Part print with two shaded views. Sizes in mm from the minimum x, y, z corner. Give positions to 0.01 mm unless a question says otherwise; leave off trailing zeros. Order: outer loops, then holes, each group sorted by start corner. A loop starts at its lowest first (then second) coordinate and runs counter-clockwise, first axis right, second up. Notation, with made-up numbers: M 41,3.5 L 46,3.5 A26 cw 46,24.5 Z; hole C -22,19.25 d4. An arc over 180 degrees is marked long. Return JSON: item names as keys, results as strings.
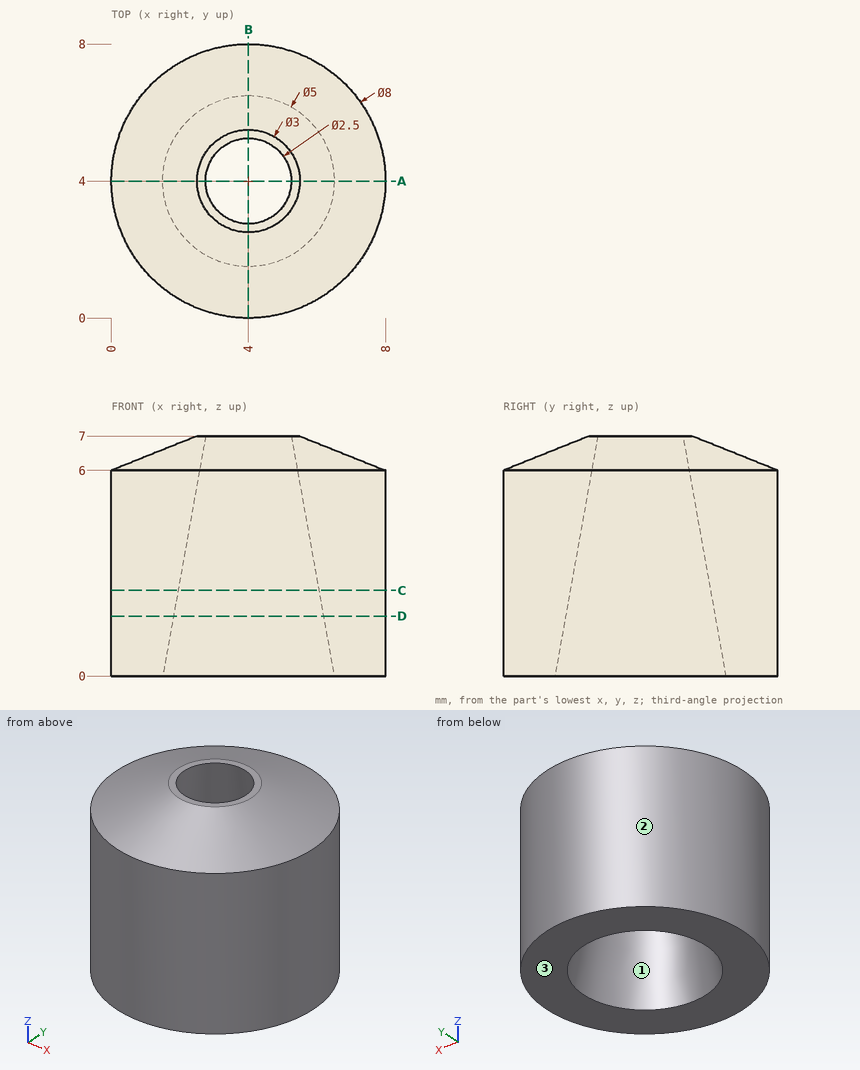
Q1. Two-plate mould, pull along Y, no slides. Class the marked faces 1, 2 and 3: +Y half, -Y half, draft (parallel to the pull), parting line (faces both ways), or undercut.
Established:
{"face 1": "undercut", "face 2": "parting line", "face 3": "draft"}
Q2. Band-saw the part on A-A (y = 4). Give the cut face in (x, z), then the cut area to 4 significant figures.
Established:
{"outline": "M 0,0 L 1.5,0 L 2.75,7 L 2.5,7 L 0,6 Z; M 5.25,7 L 6.5,0 L 8,0 L 8,6 L 5.5,7 Z", "area": "27.25 mm²"}
Q3. Probe line 1 along Y through (x, z) = (5, 3.5); line 2 along Y through (x, z) = (4.5, 2.75); line 3 along X through (y, z) = (3.5, 4). List the from-to ranges inside material, lowest first.
Established:
{"line 1": "y = 0.13 to 2.41, 5.59 to 7.87", "line 2": "y = 0.03 to 2.05, 5.95 to 7.97", "line 3": "x = 0.03 to 2.29, 5.71 to 7.97"}
Q4. Band-saw the part on C-C (z = 2.5). Give the cut face in (x, y).
Established:
{"outline": "C 4,4 d8; hole C 4,4 d4.11"}
Q5. Pin check, flat tips, straight feed: pin 1 (3 mm diameter, centred on x = 7, y = 1, fed in from -Z); pin 2 (3 mm diameter, centred on x = 6, z = 2, fed in from +Y); pin 3 (2 mm diameter, centred on y = 6.5, z = 3, fed in from -X); pin 4 (1 mm diameter, centred on x = 6, y = 6.5, fed in from +Z). Stop position of each tip, or through.
Established:
{"pin 1": "stops at z = 0", "pin 2": "stops at y = 7.97", "pin 3": "stops at x = 0.29", "pin 4": "stops at z = 6.52"}
Q6. Band-saw the part on D-D (z = 1.75). Give the cut face in (x, y) (1 decimal), then the cut area to 3 significant figures.
Established:
{"outline": "C 4,4 d8; hole C 4,4 d4.4", "area": "35.2 mm²"}
